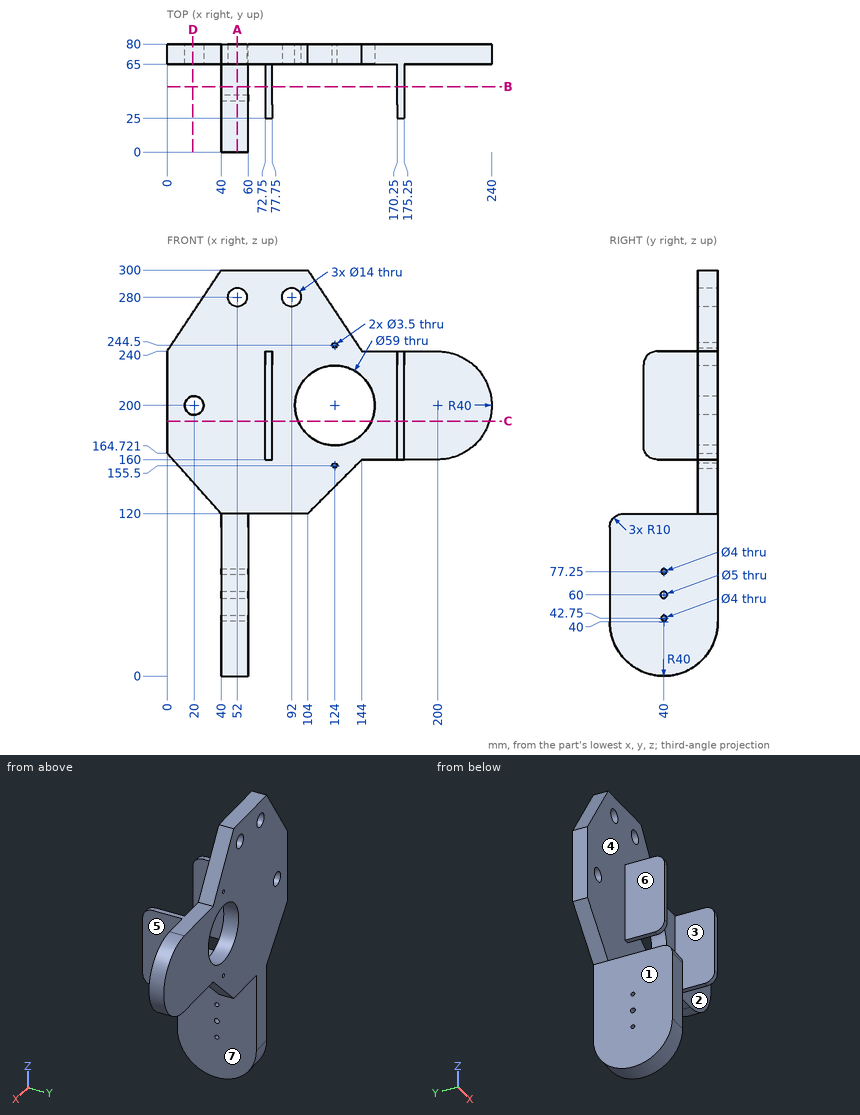
Print and shaded views of the part. All mm, measured from the part's lowest x, y and z. A direction names the side the tool comes from. Coordinates: 2 decimals unless noted, no trailing zeros. Order: outer loops, then holes, each group sorted by start corner. A loop starts at its lowest first (then second) coordinate and runs counter-clockwise, first axis right, second up. Notation, with made-up numbers: (18, 32.5) -> (57, 32.5) arc R16 ccw to (57, 58.5) -> close; hole circle Ø7 at (-1, -37). An arc over 180 degrees is marked (long way). Answer as a JSON object with one key per item and string values. Group by question number.
1) Flat gauge pins, fed straight in: pin 1 (16 mm diameter, centred on x = 52, z = 280, fed in from -Y); pin 2 (3 mm diameter, centred on y = 34, z = 52, fed in from +X); pin 3 (20 mm diameter, centred on y = 37.5, z = 205.5, fed in from -X). Where does each tip first touch, or does it go through?
2) Drill centre lines: L1, parallel to Z at x = 49.75, y = 40; L2, parallel to Z at x = 124, y = 73; L3, parallel to X at y = 71.5, z = 200. Where is each one in solid material? Low to high.
3) Pull direction X, two halves, no side cores. Call the marked faces 1, 2, 3 and 4: +X half, -X half, draft (parallel to the pull), parting line (faces both ways), or undercut.
4) Cut at C-C, the plane z = 188.5. Write the cut outline in (x, y).
5) Which spindle directions (+Z, -Z, +X, -X, +Y, -Y) get a long thin tool onto all of the face, cutting with end or side? Do the marked faces 5, 6 and 7. Say none if no direction does.
6) Cut at D-D, the plane x = 19. Write the cut outline in (y, z), then the cut area to 3 significant figures.
7) Cut at A-A, the plane x = 52. Write the cut outline in (y, z).
8) Cut at B-B, the plane y = 48.5. Write the cut outline in (x, z), then the cut area to 3 significant figures.
Check values:
{
 "1": {"pin 1": "stops at y = 65", "pin 2": "stops at x = 60", "pin 3": "stops at x = 72.75"},
 "2": {"L1": "z = 0 to 40.75, 44.75 to 57.5, 62.5 to 75.25, 79.25 to 120", "L2": "z = 140 to 153.75, 157.25 to 170.5, 229.5 to 242.75, 246.25 to 270", "L3": "x = 0 to 13, 27 to 94.5, 153.5 to 240"},
 "3": {"face 1": "-X half", "face 2": "draft", "face 3": "undercut", "face 4": "undercut"},
 "4": {"outline": "(0, 65) -> (72.75, 65) -> (72.75, 25) -> (77.75, 25) -> (77.75, 65) -> (96.83, 65) -> (96.83, 80) -> (0, 80) -> close; (151.17, 65) -> (170.25, 65) -> (170.25, 25) -> (175.25, 25) -> (175.25, 65) -> (238.31, 65) -> (238.31, 80) -> (151.17, 80) -> close"},
 "5": {"face 5": "+Z, -Z, +X, -Y", "face 6": "+Z, -Z, -X, -Y", "face 7": "-Z, +X, +Y, -Y"},
 "6": {"outline": "(65, 143.48) -> (80, 143.48) -> (80, 193.07) -> (65, 193.07) -> close; (65, 206.93) -> (80, 206.93) -> (80, 268.5) -> (65, 268.5) -> close", "area": "1,670 mm²"},
 "7": {"outline": "(0, 40) arc R40 ccw to (80, 40) -> (80, 273) -> (65, 273) -> (65, 120) -> (10, 120) arc R10 ccw to (0, 110) -> close; (65, 287) -> (80, 287) -> (80, 300) -> (65, 300) -> close; hole circle Ø5 at (40, 60); hole circle Ø4 at (40, 42.75); hole circle Ø4 at (40, 77.25)"},
 "8": {"outline": "(40, 0.91) -> (60, 0.91) -> (60, 120) -> (40, 120) -> close; (72.75, 160) -> (77.75, 160) -> (77.75, 240) -> (72.75, 240) -> close; (170.25, 160) -> (175.25, 160) -> (175.25, 240) -> (170.25, 240) -> close", "area": "3,180 mm²"}
}
